```python
from build123d import *

# Parameters (mm, degrees)
F0_W           = 85.852
F0_H           = 50.8
F1_DEPTH       = 12.7
F3_D           = 7.9248
F3_CBORE_D     = 12.7
F3_CBORE_DEPTH = 6.096
F5_DEPTH       = 50.8
F7_DEPTH       = 25.4
F9_DEPTH       = 12.7
F10_W          = 50.8
F10_H          = 47.481018
F11_DEPTH      = 12.7
F13_DEPTH      = 66.290802


with BuildPart() as f1:
    # F0 (on Top) → F1 (new body)
    with BuildSketch(Plane.XY):
        with Locations((42.926, 25.4)):
            Rectangle(F0_W, F0_H)
    extrude(amount=-F1_DEPTH)

    # F3 (through all)
    with Locations(Plane(origin=(0, 0, -12.7), x_dir=(1, 0, 0), z_dir=(0, 0, -1))):
        with Locations((69.596, -12.7), (15.748, -12.7), (15.748, -38.1), (69.596, -38.1)):
            CounterBoreHole(F3_D / 2, F3_CBORE_D / 2, F3_CBORE_DEPTH)

    # F4 (on Front) → F5 (join)
    with BuildSketch(Plane.XZ):
        Polygon((85.852, 0), (85.852, -12.7), (131.338123, -58.186123), (139.953232, -49.571014), (90.382218, 0), align=None)
    extrude(amount=-F5_DEPTH)

    # F6 (on face) → F7 (cut)
    with BuildSketch(Plane(origin=(45.191109, 0, 45.191109), x_dir=(0, 1, 0), z_dir=(0.707107, 0, 0.707107))):
        with BuildLine():
            ThreePointArc((50.8, -127.646898), (38.492922, -132.397886), (25.4, -134.01388))
            Line((25.4, -134.01388), (50.8, -134.01388))
            Line((50.8, -134.01388), (50.8, -127.646898))
        make_face()
        with BuildLine():
            Line((0, -134.01388), (25.4, -134.01388))
            ThreePointArc((25.4, -134.01388), (12.307078, -132.397886), (0, -127.646898))
            Line((0, -127.646898), (0, -134.01388))
        make_face()
    extrude(amount=-F7_DEPTH, mode=Mode.SUBTRACT)

    # F8 (on face) → F9 (join)
    with BuildSketch(Plane(origin=(45.191109, 0, 45.191109), x_dir=(0, 1, 0), z_dir=(0.707107, 0, 0.707107))):
        with BuildLine():
            Line((50.8, -127.646898), (0, -127.646898))
            ThreePointArc((0, -127.646898), (12.307078, -132.397886), (25.4, -134.01388))
            ThreePointArc((25.4, -134.01388), (38.492922, -132.397886), (50.8, -127.646898))
        make_face()
    extrude(amount=F9_DEPTH)

    # F10 (on face) → F11 (join)
    with BuildSketch(Plane(origin=(45.191109, 0, 45.191109), x_dir=(0, 1, 0), z_dir=(0.707107, 0, 0.707107))):
        with Locations((25.4, -103.906389)):
            Rectangle(F10_W, F10_H)
    extrude(amount=F11_DEPTH)

    # F12 (on face) → F13 (cut, through all)
    with BuildSketch(Plane(origin=(56.685837, 0, -56.685837), x_dir=(0.707107, 0, 0.707107), z_dir=(-0.707107, 0, 0.707107))):
        Polygon((76.60988, 15.748), (76.60988, 35.052), (70.51388, 35.052), (70.51388, 41.148), (63.90988, 41.148), (63.90988, 9.652), (70.51388, 9.652), (70.51388, 15.748), align=None)
    extrude(amount=-F13_DEPTH, mode=Mode.SUBTRACT)


solid = f1.part
```
The listing builds one solid part. Answer for the finished solid, in the listing's coordinates (mm). A direction names the side the tool comes from. Give positions to 0.01 mm unless a question says otherwise; leave off trailing zeros. Order: outer loops, then holes, each group sorted by start corner. A loop starts at its lowest first (then second) coordinate and runs counter-clockwise, first axis right, second up. Notation, with made-up numbers: (55.5, -15.75) - (90.5, -15.75) arc R11 ccw to (90.5, 3.25) - close; hole circle Ø8 at (-4.5, 34.25). An arc over 180 degrees is marked (long way). Answer in a Markdown table with one row per item. Add a question column.
Q1. Find the intervals of material crossed by line 1 along X through (y, z) = (38, -9); line 2 along X through (y, z) = (35, -2.5); line 3 along X through (y, z) = (38.1, -3.75), in increasing order. Write a range as [from, to].
Q2. For a pull along X with two mould halves and no side action, classify faces 1 (the flat face through (129.32, 42.82, -20.98)), 2 (the cylindrical face through (73.555, 12.526, -3.256)), 3 (the flat face through (42, 26, -12.7)) as released by +X, released by -X, zero draft, split by the parting line, or undercut.
Q3. The part is cut by section B-B (x = 84). Determine the outline of the cut face in (y, z).
Q4. The part is cut by section D-D (x = 116). Determine the outline of the cut face in (y, z), then the cut area to 3 significant figures.
Q5. The part is cut by section C-C (z = -25.5). Determine the outline of the cut face in (x, y).
Q6. Given P1, Ø4, axis at x = 15.5, y = 39.5, coming from the -Z side; P2, Ø10, axis at x = 65.5, y = 24, coming from the -Z side; P3, Ø5, axis at x = 128, y = 32, coming from the -Z side; P4, Ø5, axis at y = 21, z = -46.5, coming from the -X side, each flat-ended and moving along its own axis, determine where each tip first touches the part or whether it passes through.
Q7. Which of the six approach directions +Z, -Z, +X, -X, +Y, -Y give full straight-line access (tool end or side, diameter ignored) to faces 4 (the flat face through (127, 15.748, -23)), 5 (the flat face through (125.01, 12.66, -25.29)), 6 (the flat face through (96.21, 25.04, -5.83)), 7 (the flat face through (15.66, 42.24, -6.604))?
Q8. The part is cut by section A-A (y = 12.7). Determine the outline of the cut face in (x, z) (3 decimals).
Determined:
| question | item | result |
|---|---|---|
| 1 | line 1 | x = [0, 9.4], [22.1, 63.25], [75.95, 99.38], [108.72, 117.34] |
| 1 | line 2 | x = [0, 13.28], [18.22, 67.13], [72.06, 92.88] |
| 1 | line 3 | x = [0, 11.79], [19.71, 65.63], [73.56, 94.13], [109.62, 112.09] |
| 2 | face 1 | released by +X |
| 2 | face 2 | undercut |
| 2 | face 3 | zero draft |
| 3 | outline | (0, -12.7) - (50.8, -12.7) - (50.8, 0) - (0, 0) - close |
| 4 | outline | (0, -42.85) - (50.8, -42.85) - (50.8, -7.66) - (35.05, -7.66) - (35.05, -16.28) - (41.15, -16.28) - (41.15, -25.62) - (9.65, -25.62) - (9.65, -16.28) - (15.75, -16.28) - (15.75, -7.66) - (0, -7.66) - close |
| 4 | area | 1,330 mm² |
| 5 | outline | (98.65, 0) - (133.84, 0) - (133.84, 15.75) - (125.22, 15.75) - (125.22, 9.65) - (115.88, 9.65) - (115.88, 41.15) - (125.22, 41.15) - (125.22, 35.05) - (133.84, 35.05) - (133.84, 50.8) - (98.65, 50.8) - close |
| 6 | P1 | passes through |
| 6 | P2 | stops at z = -12.7 |
| 6 | P3 | stops at z = -57.35 |
| 6 | P4 | stops at x = 117.15 |
| 7 | face 4 | +Z, +X |
| 7 | face 5 | none |
| 7 | face 6 | +Z, +Y, -Y |
| 7 | face 7 | -Z |
| 8 | outline | (0, -12.7) - (9.398, -12.7) - (9.398, -6.604) - (11.786, -6.604) - (11.786, 0) - (0, 0) - close; (19.71, -6.604) - (22.098, -6.604) - (22.098, -12.7) - (63.246, -12.7) - (63.246, -6.604) - (65.634, -6.604) - (65.634, 0) - (19.71, 0) - close; (73.558, -6.604) - (75.946, -6.604) - (75.946, -12.7) - (85.852, -12.7) - (130.264, -57.112) - (138.879, -48.497) - (90.382, 0) - (73.558, 0) - close; (106.547, -6.825) - (143.549, -43.827) - (147.859, -39.517) - (110.857, -2.514) - close |
